Can you work these out from the drawing? Everything is in mm from the part's minimum corner. Coordinates: 2 decimals unless noted, no trailing zeros. Loops run counter-clockwise (first coordinate to the right, second up) from the corner with the lowest first, then second, coordinate; pieces in that order, holes last.
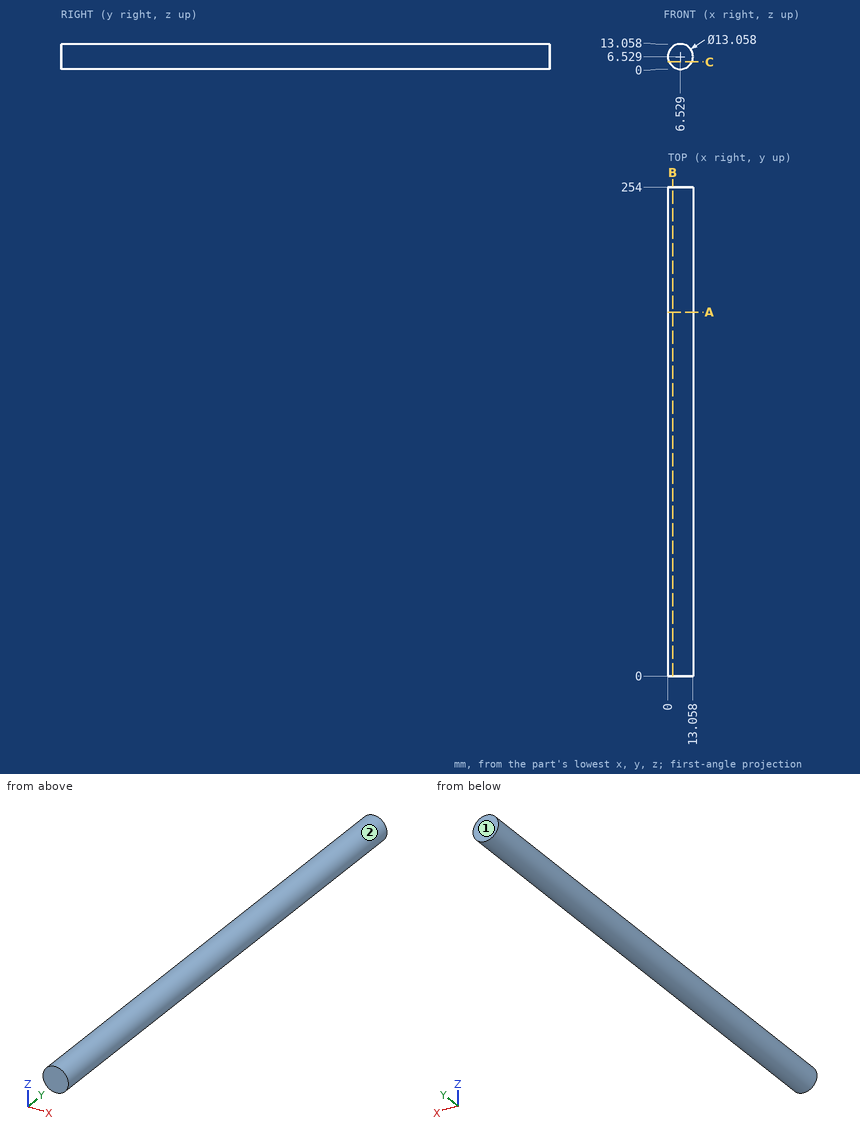
1. I need wall thicknesses on line 1 along X through (y, z) = (132.5, 6); line 2 along Z through (x, y) = (12, 158) (1 decimal). Which ranges of each line are inside material? Lowest first, please.
2. I want a section at A-A (y = 189). Please give me the cut outline in (x, z), then the cut area to 3 significant figures.
3. I want a section at C-C (z = 3.75). Please give me the cut outline in (x, y), then the cut area to 3 significant figures.
4. For pin 1 (3 mm diameter, centred on y = 225, z = 4, fed in from -X); pin 2 (6 mm diameter, centred on x = 5, y = 212.5, fed in from +Z), each with a flat end and sliding along its axis, tell me the tip position at first contact or that it passes through.
5. We'd pull the mould along X, two halves only. Please class the marked faces 1 and 2: +X half, -X half, draft (parallel to the pull), parting line (faces both ways), or undercut.
6. I want a section at B-B (x = 2.5). Please give me the cut outline in (y, z).
Response values:
1. line 1: x = 0.02 to 13.04
1. line 2: z = 3 to 10.1
2. outline: circle Ø13.06 at (6.53, 6.53)
2. area: 134 mm2
3. outline: (0.62, 0) - (12.44, 0) - (12.44, 254) - (0.62, 254) - close
3. area: 3,000 mm2
4. pin 1: stops at x = 0.08
4. pin 2: stops at z = 13.06
5. face 1: draft
5. face 2: parting line
6. outline: (0, 1.39) - (254, 1.39) - (254, 11.67) - (0, 11.67) - close
